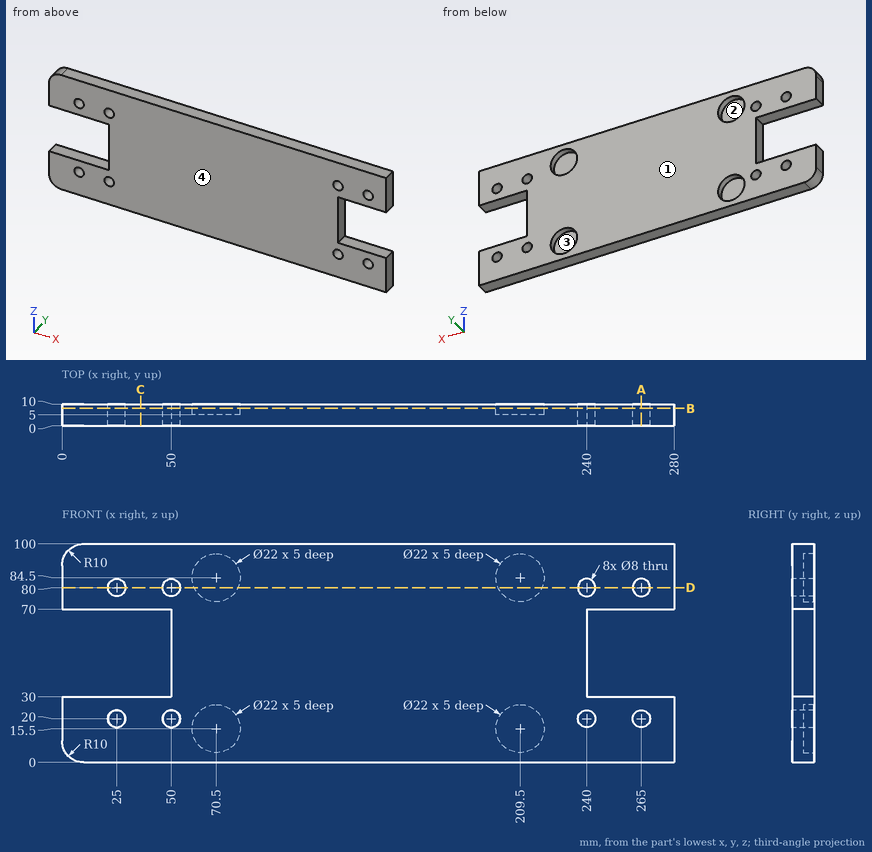
Input: dimensioned drawing with shaded views. Units: mm. Origin: part minimum x, y, z. A direction names the side the tool comes from. Give positions to 0.01 mm unless a question says otherwise; leave off trailing zeros. Loops run counter-clockwise (first coordinate to the right, second up) from the corner with the lowest first, then second, coordinate; pieces in that order, holes last. Notation, with made-up numbers: M 0.5,76 L 40.5,76 A8 ccw 40.5,82 Z; hole C -1.5,1 d11. An arc over 180 degrees is marked long. Put each result on its own line as item: value.
1) Reachability of the marked faces 3 and 4 from +Z, -Z, +X, -X, +Y, -Y: full face, straight path, thin tool, end or side. Return the list, or none.
Computed values:
face 3: +Y
face 4: +Z, -Z, +X, -X, -Y
2) Material intervals for L1, parallel to X at y = 1.25, z = 79.5; L2, parallel to X at y = 8.5, z = 84.5; L3, parallel to Z at x = 265, y = 3.25, sorted ascending. Write a range as from..to.
Computed values:
L1: x = 0..21.03, 28.97..46.03, 53.97..236.03, 243.97..261.03, 268.97..280
L2: x = 0..59.5, 81.5..198.5, 220.5..280
L3: z = 0..16, 24..30, 70..76, 84..100
3) Cut plane C-C, the plane x = 36. Return the cut outline in (y, z), plus the area to 3 significant figures.
Computed values:
outline: M 0,0 L 10,0 L 10,30 L 0,30 Z; M 0,70 L 10,70 L 10,100 L 0,100 Z
area: 600 mm^2
4) First-contact query: P1, Ø5, axis at x = 84.5, y = 6, coming from the -Z side; P2, Ø1, axis at y = 6, z = 62.5, coming from the +X side; P3, Ø11, axis at x = 213.5, z = 86, coming from the +Y side. Flat tips, straight axial feed; report the tip coordinate or a pass-through.
Computed values:
P1: stops at z = 0
P2: stops at x = 240
P3: stops at y = 5
5) Mould query, pull axis Z, two halves, no side actions, for the marked faces 1 and 2. Classes: released by +Z, released by -Z, zero draft, split by the parting line, or undercut.
Computed values:
face 1: zero draft
face 2: undercut
6) Cut plane D-D, the plane z = 80. Return the cut outline in (x, y).
Computed values:
outline: M 0,0 L 21,0 L 21,10 L 0,10 Z; M 29,0 L 46,0 L 46,10 L 29,10 Z; M 54,0 L 236,0 L 236,10 L 219.54,10 L 219.54,5 L 199.46,5 L 199.46,10 L 80.54,10 L 80.54,5 L 60.46,5 L 60.46,10 L 54,10 Z; M 244,0 L 261,0 L 261,10 L 244,10 Z; M 269,0 L 280,0 L 280,10 L 269,10 Z
7) Cut plane B-B, the plane y = 8. Give the number of separate pieces and of enclosed holes in the cut face, plus the area to 3 significant figures.
Computed values:
separate pieces: 1
enclosed holes: 12
area: 22,400 mm^2
8) Cut plane A-A, the plane x = 265. Return the cut outline in (y, z), plus the area to 3 significant figures.
Computed values:
outline: M 0,0 L 10,0 L 10,16 L 0,16 Z; M 0,24 L 10,24 L 10,30 L 0,30 Z; M 0,70 L 10,70 L 10,76 L 0,76 Z; M 0,84 L 10,84 L 10,100 L 0,100 Z
area: 440 mm^2
